Verification items for the finished model (mm, model axes). Face numbers are marked on the shaded views. A direction names the side the tool comes from. Round coordinates to 2 decimals unless told otherwise and drop trailing zeros. Order: outer loops, then holes, each group sorted by start corner. A loop starts at its lowest first (then second) coordinate and runs counter-clockwise, first axis right, second up. Notation, with made-up numbers: M -2.75,44.25 L 39.25,44.25 A24 cw 39.25,65.25 Z; hole C -37,54.25 d4. An arc over 180 degrees is marked long. Use one line per item in the form item = value. Start each with the question number.
Item 1: Tool access check on the marked faces 1, 2 and 3. Record the directions out of +Z, -Z, +X, -X, +Y, -Y that give a thin tool (end or side, any length) a straight path to the whole face; none if there is none.
Item 2: Thickness scan on probe 1 along X at (y, z) = (-0.25, 2); probe 2 along Y at (x, z) = (2.5, 3.75); probe 3 along Z at (x, y) = (-0.25, -1.75). Record the ranges inside material, lowest first. Write a range as [from, to].
Item 3: Go/stop test with flat-tipped pins: pin 1 Ø0.8 at (y, z) = (-7, 2.5) entering from -X; pin 2 Ø7 at (x, y) = (1, 3.5) entering from +Z; pin 3 Ø0.5 at (y, z) = (7.5, 2.5) entering from -X. Record where each tip stops, or that it passes through.
Item 4: Cross-section at A-A on z = 2.5. Enter the section's corners in (x, y).
Item 5: Cross-section at C-C on z = -1.5. Enter the section's corners in (x, y).
Item 6: Cross-section at B-B on x = 0. Enter the section's corners in (y, z), then the cut area to 3 significant figures.
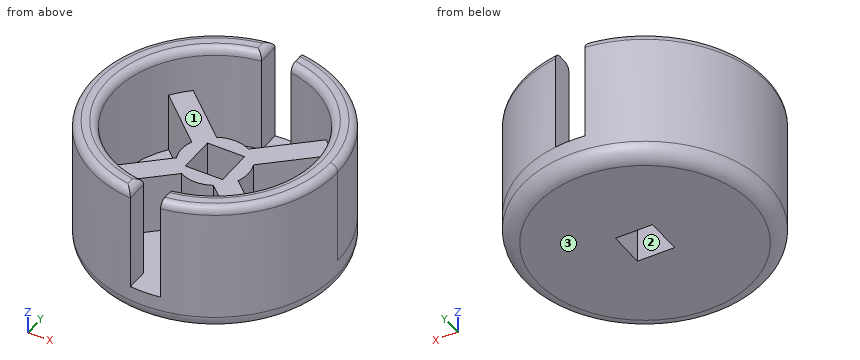
from build123d import *

# Parameters (mm, degrees)
SKETCH_1_R          = 8.25
SKETCH_1_R_2        = 6.75
EXTRUDE_1_DEPTH     = 7
EXTRUDE_START       = 2
SKETCH_2_R          = 8.25
EXTRUDE_1_2_DEPTH   = 2
EXTRUDE_3_DEPTH     = 4
SKETCH_3_W          = 2.5
SKETCH_3_H          = 2.5
CUT_EXTRUDE_1_DEPTH = 15.735162028
SKETCH_6_W          = 2
SKETCH_6_H          = 3.283082556
SKETCH_6_H_2        = 3.547491889
CUT_EXTRUDE_2_DEPTH = 7
FILLET_1_R          = 1
FILLET_2_R          = 0.5


with BuildPart() as part:
    # Эскиз1 → Extrude 1 (new body)
    with BuildSketch(Plane.XY):
        Circle(SKETCH_1_R)
        Circle(SKETCH_1_R_2, mode=Mode.SUBTRACT)
    extrude(amount=EXTRUDE_1_DEPTH)

    # Эскиз2 → Extrude 1 2 (add)
    with BuildSketch(Plane(origin=(0, 0, 0), x_dir=(-1, 0, 0), z_dir=(0, 0, -1)).offset(EXTRUDE_START)):
        Circle(SKETCH_2_R)
    extrude(amount=-EXTRUDE_1_2_DEPTH)

    # Эскиз4 → Бобышка-Вытянуть3 (add)
    with BuildSketch(Plane.XY):
        with BuildLine():
            Line((2.07406055, -0.872222927), (5.968591922, -4.413472559))
            Line((5.968591922, -4.413472559), (4.959463137, -5.523273935))
            Line((4.959463137, -5.523273935), (1.064931765, -1.982024303))
            ThreePointArc((1.064931765, -1.982024303), (-0.012257169, -2.249966613), (-1.08646291, -1.970304125))
            Line((-1.08646291, -1.970304125), (-4.961140395, -5.41713434))
            Line((-4.961140395, -5.41713434), (-5.958117889, -4.296404276))
            Line((-5.958117889, -4.296404276), (-2.083440404, -0.849574061))
            ThreePointArc((-2.083440404, -0.849574061), (-2.249966613, 0.012257169), (-2.07406055, 0.872222927))
            Line((-2.07406055, 0.872222927), (-5.968591922, 4.413472559))
            Line((-5.968591922, 4.413472559), (-4.959463137, 5.523273935))
            Line((-4.959463137, 5.523273935), (-1.064931765, 1.982024303))
            ThreePointArc((-1.064931765, 1.982024303), (0.012257169, 2.249966613), (1.08646291, 1.970304125))
            Line((1.08646291, 1.970304125), (4.961140395, 5.41713434))
            Line((4.961140395, 5.41713434), (5.958117889, 4.296404276))
            Line((5.958117889, 4.296404276), (2.083440404, 0.849574061))
            ThreePointArc((2.083440404, 0.849574061), (2.249966613, -0.012257169), (2.07406055, -0.872222927))
        make_face()
    extrude(amount=EXTRUDE_3_DEPTH)

    # Эскиз3 → Вырез-Вытянуть1 (cut, through all)
    with BuildSketch(Plane(origin=(0, 0, -2), x_dir=(-1, 0, 0), z_dir=(0, 0, -1))):
        Rectangle(SKETCH_3_W, SKETCH_3_H)
    extrude(amount=-CUT_EXTRUDE_1_DEPTH, mode=Mode.SUBTRACT)

    # Эскиз6 → Вырез-Вытянуть2 (cut)
    with BuildSketch(Plane.XY.offset(7)):
        with Locations((0.173720833, 7.205154333)):
            Rectangle(SKETCH_6_W, SKETCH_6_H)
        with Locations((0.173720833, -7.513631889)):
            Rectangle(SKETCH_6_W, SKETCH_6_H_2)
    extrude(amount=-CUT_EXTRUDE_2_DEPTH, mode=Mode.SUBTRACT)

    # Скругление1
    fillet_1_edges = [part.edges().sort_by_distance(p)[0] for p in [
        (8.25, 0, -2),
    ]]
    fillet(fillet_1_edges, radius=FILLET_1_R)

    # Скругление2
    # the kernel refuses this fillet: 0.5 mm, written as the material it takes off along each edge
    with BuildSketch(Plane(origin=(0, 0, 7), x_dir=(1, 0, 0), z_dir=(0, -1, 0))) as fillet_2_piece_1:
        with BuildLine():
            CenterArc((8.25 - FILLET_2_R, -FILLET_2_R), FILLET_2_R, 0, 90)
            Line((8.25, -FILLET_2_R), (8.25, 0))
            Line((8.25, 0), (8.25 - FILLET_2_R, 0))
        make_face()
    revolve(axis=Axis((0, 0, 7), (0, 0, 1)), revolution_arc=90.504884873, mode=Mode.SUBTRACT)
    with BuildSketch(Plane(origin=(0, 0, 7), x_dir=(0.06267760440756695, 0.9980338260328296, 0), z_dir=(0.9980338260328296, -0.06267760440756695, 0))) as fillet_2_piece_2:
        with BuildLine():
            CenterArc((6.75 + FILLET_2_R, -FILLET_2_R), FILLET_2_R, 90, 90)
            Line((6.75 + FILLET_2_R, 0), (6.75, 0))
            Line((6.75, 0), (6.75, -FILLET_2_R))
        make_face()
    revolve(axis=Axis((0, 0, 7), (0, 0, 1)), revolution_arc=187.187035343, mode=Mode.SUBTRACT)
    with BuildSketch(Plane(origin=(0, 0, 7), x_dir=(-0.01064718913448663, 0.9999433170752903, 0), z_dir=(-0.9999433170752903, -0.01064718913448663, 0))) as fillet_2_piece_3:
        with BuildLine():
            CenterArc((6.75 + FILLET_2_R, FILLET_2_R), FILLET_2_R, 180, 90)
            Line((6.75 + FILLET_2_R, 0), (6.75, 0))
            Line((6.75, 0), (6.75, FILLET_2_R))
        make_face()
    revolve(axis=Axis((0, 0, 7), (0, 0, -1)), revolution_arc=181.220101055, mode=Mode.SUBTRACT)
    with BuildSketch(Plane(origin=(-0.826279167, 9.458517694, 7), x_dir=(0, 0, -1), z_dir=(0, -1, 0))) as fillet_2_piece_4:
        with BuildLine():
            CenterArc((FILLET_2_R, -FILLET_2_R), FILLET_2_R, 90, 90)
            Line((0, -FILLET_2_R), (0, 0))
            Line((0, 0), (FILLET_2_R, 0))
        make_face()
    extrude(amount=4.009281713, mode=Mode.SUBTRACT)
    with BuildSketch(Plane(origin=(-0.826279167, -5.449235982, 7), x_dir=(-1, 0, 0), z_dir=(0, -1, 0))) as fillet_2_piece_5:
        with BuildLine():
            CenterArc((FILLET_2_R, FILLET_2_R), FILLET_2_R, 180, 90)
            Line((0, FILLET_2_R), (0, 0))
            Line((0, 0), (FILLET_2_R, 0))
        make_face()
    extrude(amount=4.009281713, mode=Mode.SUBTRACT)
    with BuildSketch(Plane(origin=(0, 0, 7), x_dir=(0.05138276513110792, 0.9986790332471597, 0), z_dir=(0.9986790332471597, -0.05138276513110792, 0))) as fillet_2_piece_6:
        with BuildLine():
            CenterArc((8.25 - FILLET_2_R, -FILLET_2_R), FILLET_2_R, 0, 90)
            Line((8.25 - FILLET_2_R, 0), (8.25, 0))
            Line((8.25, 0), (8.25, -FILLET_2_R))
        make_face()
    revolve(axis=Axis((0, 0, 7), (0, 0, 1)), revolution_arc=185.890625165, mode=Mode.SUBTRACT)
    with BuildSketch(Plane(origin=(0, 0, 7), x_dir=(-0.008811789331912054, -0.9999611754307114, 0), z_dir=(-0.9999611754307114, 0.008811789331912054, 0))) as fillet_2_piece_7:
        with BuildLine():
            CenterArc((8.25 - FILLET_2_R, -FILLET_2_R), FILLET_2_R, 0, 90)
            Line((8.25 - FILLET_2_R, 0), (8.25, 0))
            Line((8.25, 0), (8.25, -FILLET_2_R))
        make_face()
    revolve(axis=Axis((0, 0, 7), (0, 0, 1)), revolution_arc=90.504884873, mode=Mode.SUBTRACT)


solid = part.part
Output values:
q1.face_1 = +Z
q1.face_2 = +Z, -Z
q1.face_3 = -Z, +X, -X, +Y, -Y
q2.probe_1 = [-8.25, -6.75], [-2.24, -1.25], [1.25, 2.24], [6.75, 8.25]
q2.probe_2 = [-7.86, -6.27], [-3.29, -1.26], [1.22, 3.23], [6.27, 7.86]
q2.probe_3 = [-2, 4]
q3.pin_1 = -4.95
q3.pin_2 = 6.99
q3.pin_3 = -3.94
q4.outline = M -4.51,-5.02 L -1.09,-1.97 A2.25 ccw 1.06,-1.98 L 4.46,-5.07 A6.75 cw 1.17,-6.65 L 1.17,-8.17 A8.25 ccw 1.17,8.17 L 1.17,6.65 A6.75 cw 4.51,5.02 L 1.09,1.97 A2.25 ccw -1.06,1.98 L -4.46,5.07 A6.75 cw -0.83,6.7 L -0.83,8.21 A8.25 ccw -0.83,-8.21 L -0.83,-6.7 A6.75 cw Z; hole M -5.51,-3.9 L -2.08,-0.85 A2.25 cw -2.07,0.87 L -5.47,3.96 A6.75 ccw Z; hole M -1.25,-1.25 L 1.25,-1.25 L 1.25,1.25 L -1.25,1.25 Z; hole M 2.07,-0.87 L 5.47,-3.96 A6.75 ccw 5.51,3.9 L 2.08,0.85 A2.25 cw Z
q5.outline = C 0,0 d16.23; hole M -1.25,-1.25 L 1.25,-1.25 L 1.25,1.25 L -1.25,1.25 Z
q6.outline = M -8.25,-1 A1 ccw -7.25,-2 L -1.25,-2 L -1.25,4 L -2.25,4 L -2.25,0 L -8.25,0 Z; M 1.25,-2 L 7.25,-2 A1 ccw 8.25,-1 L 8.25,0 L 2.25,0 L 2.25,4 L 1.25,4 Z
q6.area = 35.6 mm2
